Check sheet for the modelled part. Datum: model origin and axes. Units: mm. Face numbers are marked on the shaded views. A direction names the side the tool comes from. Round coordinates to 2 decimals unless told otherwise and drop trailing zeros. Order: outer loops, then holes, each group sorted by start corner. A loop starts at its lowest first (then second) coordinate and runs counter-clockwise, first axis right, second up. Notation, with made-up numbers: (43, 46.5) -> (72, 46.5) arc R8 ccw to (72, 54.5) -> close; hole circle Ø9 at (89.25, 42.25). An arc over 180 degrees is marked (long way). Use CSV: the item, a comma, the result in double quotes.
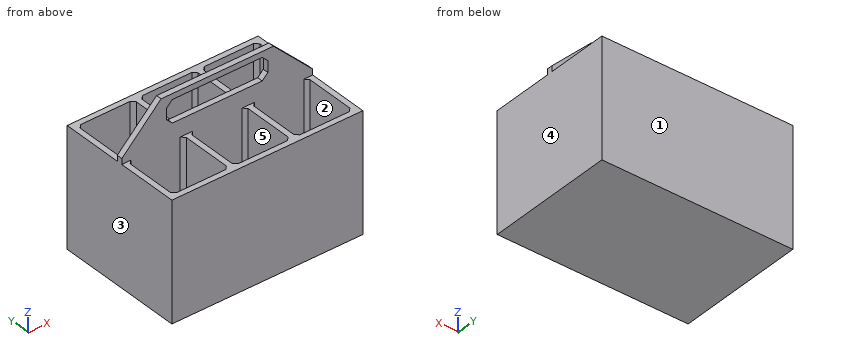
Autodesk Fusion 360 part; units mm, degrees
sketch "Sketch1" plane through (0, 0, 0) normal (0, 0, 1) x (1, 0, 0)
  line L0 (0, 0) -> (5, 0)
  line L1 (5, 0) -> (5, 5)
  line L2 (5, 5) -> (0, 5)
  line L3 (0, 5) -> (0, 0)
  line L4 (5, 5) -> (5.5, 5) construction
  line L5 (5.5, 5) -> (10.5, 5)
  line L6 (10.5, 5) -> (10.5, 0)
  line L7 (10.5, 0) -> (5.5, 0)
  line L8 (5.5, 0) -> (5.5, 5)
  line L9 (10.5, 5) -> (11, 5) construction
  line L10 (11, 5) -> (16, 5)
  line L11 (16, 5) -> (16, 0)
  line L12 (16, 0) -> (11, 0)
  line L13 (11, 0) -> (11, 5)
  line L14 (0, 5) -> (0, 5.5) construction
  line L15 (0, 5.25) -> (16.5, 5.25) construction
  line L16 (16, 10.5) -> (11, 10.5)
  line L17 (16, 5.5) -> (16, 10.5)
  line L18 (11, 5.5) -> (16, 5.5)
  line L19 (11, 10.5) -> (11, 5.5)
  line L20 (10.5, 5.5) -> (10.5, 10.5)
  line L21 (5.5, 5.5) -> (10.5, 5.5)
  line L22 (10.5, 10.5) -> (5.5, 10.5)
  line L23 (5.5, 10.5) -> (5.5, 5.5)
  line L24 (5, 10.5) -> (5, 5.5)
  line L25 (0, 10.5) -> (5, 10.5)
  line L26 (5, 5.5) -> (0, 5.5)
  line L27 (0, 5.5) -> (0, 10.5)
  line L28 (0, 10.5) -> (-0.5, 10.5) construction
  line L29 (-0.5, 10.5) -> (-0.5, 11) construction
  line L30 (-0.5, 11) -> (16.5, 11)
  line L31 (16.5, 11) -> (16.5, -0.5)
  line L32 (16.5, -0.5) -> (-0.5, -0.5)
  line L33 (-0.5, -0.5) -> (-0.5, 11)
  dimension "d1" = 5
  dimension "d2" = 5
  dimension "d3" = 0.5
  dimension "d4" = 5
  dimension "d5" = 5
  dimension "d6" = 5
  dimension "d7" = 0.5
  dimension "d8" = 0.5
  dimension "d9" = 0.5
  dimension "d10" = 0.5
  dimension "d11" = 17
  dimension "d12" = 11.5
extrude "Extrude1" add sketch "Sketch1" along normal blind 10 makes body 1
chamfer "Chamfer1" distance 0.3 angle 45 23 edges at (0, 5, 5) (0, 10.5, 5) (5.5, 5, 5) (5.5, 10.5, 5) (11, 5, 5) (11, 10.5, 5) (0, 5.5, 5) (0, 0, 5) (5, 0, 5) (5, 5, 5) (11, 0, 5) (16, 5, 5) (16, 10.5, 5) (16, 0, 5) (10.5, 5.5, 5) (16, 5.5, 5) (10.5, 0, 5) (5, 5.5, 5) (5.5, 5.5, 5) (11, 5.5, 5) (10.5, 5, 5) (10.5, 10.5, 5) (5, 10.5, 5) on bodies 1
sketch "Sketch2" plane through (0, 0, 0) normal (0, 0, -1) x (1, 0, 0)
  line L0 (4.7, -5.5) -> (5, -5.8)
  line L1 (5, -5.8) -> (5, -10.2)
  line L2 (5, -10.2) -> (4.7, -10.5)
  line L3 (4.7, -10.5) -> (0.3, -10.5)
  line L4 (0.3, -10.5) -> (0, -10.2)
  line L5 (0, -10.2) -> (0, -5.8)
  line L6 (0, -5.8) -> (0.3, -5.5)
  line L7 (0.3, -5.5) -> (4.7, -5.5)
  line L8 (0, -0.3) -> (0.3, 0)
  line L9 (0.3, 0) -> (4.7, 0)
  line L10 (4.7, 0) -> (5, -0.3)
  line L11 (5, -0.3) -> (5, -4.7)
  line L12 (5, -4.7) -> (4.7, -5)
  line L13 (4.7, -5) -> (0.3, -5)
  line L14 (0.3, -5) -> (0, -4.7)
  line L15 (0, -4.7) -> (0, -0.3)
  line L16 (10.2, 0) -> (10.5, -0.3)
  line L17 (10.5, -0.3) -> (10.5, -4.7)
  line L18 (10.5, -4.7) -> (10.2, -5)
  line L19 (10.2, -5) -> (5.8, -5)
  line L20 (5.8, -5) -> (5.5, -4.7)
  line L21 (5.5, -4.7) -> (5.5, 0)
  line L22 (5.5, 0) -> (10.2, 0)
  line L23 (5.5, -5.8) -> (5.8, -5.5)
  line L24 (5.8, -5.5) -> (10.2, -5.5)
  line L25 (10.2, -5.5) -> (10.5, -5.8)
  line L26 (10.5, -5.8) -> (10.5, -10.2)
  line L27 (10.5, -10.2) -> (10.2, -10.5)
  line L28 (10.2, -10.5) -> (5.8, -10.5)
  line L29 (5.8, -10.5) -> (5.5, -10.2)
  line L30 (5.5, -10.2) -> (5.5, -5.8)
  line L31 (11, -5.8) -> (11.3, -5.5)
  line L32 (11.3, -5.5) -> (15.7, -5.5)
  line L33 (15.7, -5.5) -> (16, -5.8)
  line L34 (16, -5.8) -> (16, -10.2)
  line L35 (16, -10.2) -> (15.7, -10.5)
  line L36 (15.7, -10.5) -> (11.3, -10.5)
  line L37 (11.3, -10.5) -> (11, -10.2)
  line L38 (11, -10.2) -> (11, -5.8)
  line L39 (15.7, 0) -> (16, -0.3)
  line L40 (16, -0.3) -> (16, -4.7)
  line L41 (16, -4.7) -> (15.7, -5)
  line L42 (15.7, -5) -> (11.3, -5)
  line L43 (11.3, -5) -> (11, -4.7)
  line L44 (11, -4.7) -> (11, -0.3)
  line L45 (11, -0.3) -> (11.3, 0)
  line L46 (11.3, 0) -> (15.7, 0)
  line L47 (16.5, 0.5) -> (-0.5, 0.5)
  line L48 (-0.5, 0.5) -> (-0.5, -11)
  line L49 (-0.5, -11) -> (16.5, -11)
  line L50 (16.5, -11) -> (16.5, 0.5)
  line L51 (16.5, -11) -> (-0.5, -11)
  line L52 (-0.5, -11) -> (-0.5, 0.5)
  line L53 (-0.5, 0.5) -> (16.5, 0.5)
  line L54 (16.5, 0.5) -> (16.5, -11)
extrude "Extrude2" add sketch "Sketch2" along normal blind 0.5 contours L0 L1 L2 L3 L4 L5 L6 L7 | L8 L9 L10 L11 L12 L13 L14 L15 | L16 L17 L18 L19 L20 L21 L22 | L23 L24 L25 L26 L27 L28 L29 L30 | L31 L32 L33 L34 L35 L36 L37 L38 | L39 L40 L41 L42 L43 L44 L45 L46 | L47 L48 L49 L50 L51 L52 L53 L54 bodies 1
sketch "Sketch3" plane through (0, 0, 10) normal (0, 0, 1) x (-1, 0, 0)
  line L0 (-4.7, -5.5) -> (-0.3, -5.5)
  line L1 (-0.3, -5.5) -> (0, -5.8)
  line L2 (0, -5.8) -> (0, -10.2)
  line L3 (0, -10.2) -> (-0.3, -10.5)
  line L4 (-0.3, -10.5) -> (-4.7, -10.5)
  line L5 (-4.7, -10.5) -> (-5, -10.2)
  line L6 (-5, -10.2) -> (-5, -5.8)
  line L7 (-5, -5.8) -> (-4.7, -5.5)
  line L8 (0, -0.3) -> (0, -4.7)
  line L9 (0, -4.7) -> (-0.3, -5)
  line L10 (-0.3, -5) -> (-4.7, -5)
  line L11 (-4.7, -5) -> (-5, -4.7)
  line L12 (-5, -4.7) -> (-5, -0.3)
  line L13 (-5, -0.3) -> (-4.7, 0)
  line L14 (-4.7, 0) -> (-0.3, 0)
  line L15 (-0.3, 0) -> (0, -0.3)
  line L16 (-10.2, 0) -> (-5.5, 0)
  line L17 (-5.5, 0) -> (-5.5, -4.7)
  line L18 (-5.5, -4.7) -> (-5.8, -5)
  line L19 (-5.8, -5) -> (-10.2, -5)
  line L20 (-10.2, -5) -> (-10.5, -4.7)
  line L21 (-10.5, -4.7) -> (-10.5, -0.3)
  line L22 (-10.5, -0.3) -> (-10.2, 0)
  line L23 (-5.5, -5.8) -> (-5.5, -10.2)
  line L24 (-5.5, -10.2) -> (-5.8, -10.5)
  line L25 (-5.8, -10.5) -> (-10.2, -10.5)
  line L26 (-10.2, -10.5) -> (-10.5, -10.2)
  line L27 (-10.5, -10.2) -> (-10.5, -5.8)
  line L28 (-10.5, -5.8) -> (-10.2, -5.5)
  line L29 (-10.2, -5.5) -> (-5.8, -5.5)
  line L30 (-5.8, -5.5) -> (-5.5, -5.8)
  line L31 (-11, -5.8) -> (-11, -10.2)
  line L32 (-11, -10.2) -> (-11.3, -10.5)
  line L33 (-11.3, -10.5) -> (-15.7, -10.5)
  line L34 (-15.7, -10.5) -> (-16, -10.2)
  line L35 (-16, -10.2) -> (-16, -5.8)
  line L36 (-16, -5.8) -> (-15.7, -5.5)
  line L37 (-15.7, -5.5) -> (-11.3, -5.5)
  line L38 (-11.3, -5.5) -> (-11, -5.8)
  line L39 (-15.7, 0) -> (-11.3, 0)
  line L40 (-11.3, 0) -> (-11, -0.3)
  line L41 (-11, -0.3) -> (-11, -4.7)
  line L42 (-11, -4.7) -> (-11.3, -5)
  line L43 (-11.3, -5) -> (-15.7, -5)
  line L44 (-15.7, -5) -> (-16, -4.7)
  line L45 (-16, -4.7) -> (-16, -0.3)
  line L46 (-16, -0.3) -> (-15.7, 0)
  line L47 (0.5, 0.5) -> (-16.5, 0.5)
  line L48 (-16.5, 0.5) -> (-16.5, -11)
  line L49 (-16.5, -11) -> (0.5, -11)
  line L50 (0.5, -11) -> (0.5, 0.5)
  line L51 (-16.5, -5) -> (0.5, -5)
  line L52 (0.5, -5) -> (0.5, -5.5)
  line L53 (0.5, -5.5) -> (-16.5, -5.5)
  line L54 (-16.5, -5.5) -> (-16.5, -5)
  dimension "d18" = 17
  dimension "d19" = 0.5
extrude "Extrude3" add sketch "Sketch3" along normal blind 4 contours L0 L10 L19 L29 L37 L43 L48 L50 L51 L52 L53 L54 bodies 1
chamfer "Chamfer2" distance 0.3 angle 45 1 edges at (5.5, 0, 5) on bodies 1
chamfer "Chamfer3" distance 3.5 angle 45 2 edges at (16.5, 5.25, 14) (-0.5, 5.25, 14) on bodies 1
sketch "Sketch4" plane through (0, 5.5, 0) normal (0, 1, 0) x (-1, 0, 0)
  line L0 (0.5, 10.5) -> (-3, 14)
  line L1 (-3, 14) -> (-13, 14)
  line L2 (-13, 14) -> (-16.5, 10.5)
  line L3 (-16.5, 10.5) -> (-16.5, 10)
  line L4 (-16.5, 10) -> (-15.7, 10)
  line L5 (-15.7, 10) -> (-15.7, 0)
  line L6 (-15.7, 0) -> (-11.3, 0)
  line L7 (-11.3, 0) -> (-11.3, 10)
  line L8 (-11.3, 10) -> (-10.2, 10)
  line L9 (-10.2, 10) -> (-10.2, 0)
  line L10 (-10.2, 0) -> (-5.8, 0)
  line L11 (-5.8, 0) -> (-5.8, 10)
  line L12 (-5.8, 10) -> (-4.7, 10)
  line L13 (-4.7, 10) -> (-4.7, 0)
  line L14 (-4.7, 0) -> (-0.3, 0)
  line L15 (-0.3, 0) -> (-0.3, 10)
  line L16 (-0.3, 10) -> (0.5, 10)
  line L17 (0.5, 10) -> (0.5, 10.5)
  line L18 (-12.5, 13.5) -> (-3.5, 13.5)
  line L19 (-12.5, 13.5) -> (-3.5, 13.5)
  line L20 (-3.5, 13.5) -> (-3.5, 11.5)
  line L21 (-3.5, 11.5) -> (-12.5, 11.5)
  line L22 (-12.5, 11.5) -> (-12.5, 13.5)
  line L23 (-12.5, 12) -> (-12, 11.5)
  line L24 (-12.5, 13) -> (-12, 13.5)
  line L25 (-4, 13.5) -> (-3.5, 13)
  line L26 (-3.5, 12) -> (-4, 11.5)
extrude "Extrude4" cut sketch "Sketch4" against normal up to surface (0.5 mm away) contours L18 L19 L20 L21 L22 L23 L24 L25 L26 bodies 1
scale "Scale1" factor 2.352 about (16, 10.2, 10) bodies 1
copy_body "Body->Comp1" bodies 1 removing the originals makes body 2 in component "Component"
component "Component" placed x (1, 0, 0) y (0, 1, 0) z (0, 0, 1) at (0, 0, 0)
Q1. Access from +Z, -Z, +X, -X, +Y, -Y to the whole of each face (thin tool, end or side, straight path). Record for the marked faces 4 and 5.
Result sheet:
face 4,"+Z, -Z, +X, +Y, -Y"
face 5,"+Z"
Q2. Mould release check, pull along Y, two halves, no side actions. Record for the marked faces 1, 2 and 3: pulls with the +Y half, pulls with the -Y half, needs draft (parallel to the pull), parting line crosses it, or undercut.
Result sheet:
face 1,"pulls with the +Y half"
face 2,"undercut"
face 3,"needs draft"
Q3. Sectioned sample at C-C, the plane z = 0. State how many separate pieces and enclosed holes the cut face has, then the cut area to 3 significant figures.
Result sheet:
separate pieces,"1"
enclosed holes,"6"
area,"258 mm^2"
Q4. Scan lines: L1, parallel to Y at x = -0.5, z = 6; L2, parallel to X at y = 9.75, z = -12; L3, parallel to Z at x = -19, y = -7.75. Record each from-to range of solid material in increasing order.
Result sheet:
L1,"y = -14.97 to -13.79, -2.03 to -0.85, 10.91 to 12.08"
L2,"x = -22.81 to -21.63, -9.87 to -8.7, 3.06 to 4.24, 16 to 17.18"
L3,"z = -14.7 to -13.52"
Q5. Go/stop test with flat-tipped pins: pin 1 (13 mm diameter, centred on x = 12.5, y = -10.5, fed in from +Z); pin 2 (13 mm diameter, centred on x = 9.5, y = 3, fed in from +Z); pin 3 (0.6 mm diameter, centred on y = -1.5, z = 16.5, fed in from +X); pin 4 (3 mm diameter, centred on x = 10.5, y = 1.5, fed in from +Z). Record where each tip stops, or that it passes through.
Result sheet:
pin 1,"stops at z = 10"
pin 2,"stops at z = 19.41"
pin 3,"stops at x = 12.15"
pin 4,"stops at z = -13.52"
Q6. Sectioned sample at D-D, the plane z = 10.5. Enter the section's corners in (x, y).
Result sheet:
outline,"(-22.81, -2.03) -> (17.18, -2.03) -> (17.18, -0.85) -> (-22.81, -0.85) -> close"
Q7. Sectioned sample at A-A, the plane y = -4.75. Enter the section's corners in (x, z), then the cut area to 3 significant figures.
Result sheet:
outline,"(-22.81, -14.7) -> (17.18, -14.7) -> (17.18, 10) -> (16, 10) -> (16, -13.52) -> (4.24, -13.52) -> (4.24, 10) -> (3.06, 10) -> (3.06, -13.52) -> (-8.7, -13.52) -> (-8.7, 10) -> (-9.87, 10) -> (-9.87, -13.52) -> (-21.63, -13.52) -> (-21.63, 10) -> (-22.81, 10) -> close"
area,"158 mm^2"
Q8. Sectioned sample at B-B, the plane x = 13. Enter the section's corners in (y, z).
Result sheet:
outline,"(-14.97, -14.7) -> (12.08, -14.7) -> (12.08, 10) -> (10.91, 10) -> (10.91, -13.52) -> (-0.85, -13.52) -> (-0.85, 15.35) -> (-2.03, 15.35) -> (-2.03, -13.52) -> (-13.79, -13.52) -> (-13.79, 10) -> (-14.97, 10) -> close"
